The model under review builds one solid part; all positions refer to its coordinate system, in mm. A direction names the side the tool comes from. Round coordinates to 2 decimals unless told otherwise and drop trailing zeros. Write each loop counter-clockwise with the first axis right and the second up, starting at its lowest first coordinate (ties: lowest second). Pieces come first, ordered by that corner, then holes. Notation, with made-up numbers: (87, 80) - (117, 80) arc R28 cw to (117, 119) - close; hole circle Ø6 at (-32.5, 41.25). An arc over 180 degrees is marked (long way). Write each question's results on one line, items separated by ' | '.
```python
from build123d import *

# Parameters (mm, degrees)
SKETCH_1_R          = 5.5
EXTRUDE_1_DEPTH     = 37.5
SKETCH_2_R          = 4.25
CUT_EXTRUDE_1_DEPTH = 13
SKETCH_3_R          = 4.25
CUT_EXTRUDE_2_DEPTH = 101.822385015


with BuildPart() as part:
    # 草图1 → 凸台-拉伸1 (new, symmetric)
    with BuildSketch(Plane.XY):
        Polygon((0, 0), (80, 0), (80, 8), (64.335195596, 8), (51.148707324, 39.834998826), (62.225396744, 50.911688245), (56.568542495, 56.568542495), align=None)
        with Locations((22.17310878, 9.184402377)):
            Circle(SKETCH_1_R, mode=Mode.SUBTRACT)
        Polygon((7.242640687, 3), (15.457113006, 3), (13.279414953, 9.036774265), align=None, mode=Mode.SUBTRACT)
        with BuildLine():
            Line((29.347952769, 6), (61.91644612, 6))
            Line((61.91644612, 6), (48.024179606, 39.538898231))
            Line((48.024179606, 39.538898231), (24.994777104, 16.509495729))
            ThreePointArc((24.994777104, 16.509495729), (24.712781801, 15.655157608), (25.231380538, 14.919990739))
            ThreePointArc((25.231380538, 14.919990739), (28.178325742, 11.671844687), (28.391306903, 7.29125365))
            ThreePointArc((28.391306903, 7.29125365), (28.544443699, 6.404707488), (29.347952769, 6))
        make_face(mode=Mode.SUBTRACT)
    extrude(amount=EXTRUDE_1_DEPTH, both=True)

    # 草图2 → 切除-拉伸1 (cut)
    with BuildSketch(Plane(origin=(0, 0, 0), x_dir=(0, 0, 1), z_dir=(-0.7071067811865477, 0.7071067811865475, 0))):
        with Locations(Location((20, 70, 0), (0, 0, 270))):
            Circle(SKETCH_2_R)
        with Locations(Location((-20, 70, 0), (0, 0, 270))):
            Circle(SKETCH_2_R)
    extrude(amount=-CUT_EXTRUDE_1_DEPTH, mode=Mode.SUBTRACT)

    # 草图3 → 切除-拉伸2 (cut, through all)
    with BuildSketch(Plane(origin=(0, 8, 0), x_dir=(1, 0, 0), z_dir=(0, 1, 0))):
        with Locations(Location((70, -20, 0), (0, 0, 270))):
            Circle(SKETCH_3_R)
        with Locations(Location((70, 20, 0), (0, 0, 270))):
            Circle(SKETCH_3_R)
    extrude(amount=-CUT_EXTRUDE_2_DEPTH, mode=Mode.SUBTRACT)


solid = part.part
```
Q1. The part is to be moulded in two halves that separate along X. For faces 1 (the flat face through (14.38, 5.98, 0.52)), 2 (the flat face through (56.61, 45.296, 0.525)), 3 (the flat face through (34, 28, -37.5)), say which applies: released by +X, released by -X, zero draft, split by the parting line, or undercut.
Evaluation:
face 1: undercut | face 2: released by +X | face 3: zero draft
Q2. Insertion check: P1, Ø6.5, axis at x = 9.5, z = 12, coming from the +Y side; P2, Ø5, axis at x = 14, z = 1.5, coming from the +Y side; P3, Ø12, axis at y = 41, z = -10.5, coming from the +X side. Each pin has a flat end and moves straight along its axis. Give the tip position at first contact, or say it passes through.
Evaluation:
P1: stops at y = 12.75 | P2: stops at y = 16.5 | P3: stops at x = 58.31
Q3. We need section A-A (x = 70). State the section outline as (y, z) points, plus the area to 3 significant figures.
Evaluation:
outline: (0, -37.5) - (8, -37.5) - (8, -24.25) - (0, -24.25) - close; (0, -15.75) - (8, -15.75) - (8, 15.75) - (0, 15.75) - close; (0, 24.25) - (8, 24.25) - (8, 37.5) - (0, 37.5) - close | area: 464 mm^2
Q4. For probe 1 along X at (y, z) = (4.25, -20); probe 2 along Y at (x, z) = (56.5, -15); probe 3 along X at (y, z) = (5, 20), list the stretches that pass through material, from the lowest coordinate up.
Evaluation:
probe 1: x = 4.25 to 8.49, 15.01 to 19.74, 24.6 to 65.75, 74.25 to 80 | probe 2: y = 0 to 6, 19.08 to 26.92, 45.19 to 56.5 | probe 3: x = 5 to 9.24, 14.74 to 18.6, 25.74 to 65.75, 74.25 to 80
Q5. We need section C-C (y = 27.5). State the section outline as (x, z) points, plus the area to 3 significant figures.
Evaluation:
outline: (27.5, -37.5) - (35.99, -37.5) - (35.99, 37.5) - (27.5, 37.5) - close; (53.01, -37.5) - (56.26, -37.5) - (56.26, 37.5) - (53.01, 37.5) - close | area: 880 mm^2
Q6. Tool access review of faces 4 (the flat face through (80, 4, 1)), 5 (the flat face through (34, 28, 37.5)), 6 (the flat face through (72, 8, 1)), 7 (the flat face through (57.834, 23.695, 0.525)), 8 (the flat face through (11, 3, 1)): name each direction out of +Z, -Z, +X, -X, +Y, -Y from which nothing blocks a thin tool from reaching the whole face with its end or side.
Evaluation:
face 4: +Z, -Z, +X, +Y, -Y | face 5: +Z, +X, -X, +Y, -Y | face 6: +Z, -Z, +X, +Y | face 7: +Z, -Z, +X | face 8: +Z, -Z
Q7. We need section B-B (z = 20). State how many separate pieces and enclosed holes the cut face has, plus the area to 3 significant figures.
Evaluation:
separate pieces: 3 | enclosed holes: 3 | area: 873 mm^2
Q8. We need section D-D (x = 23). State the section outline as (y, z) points.
Evaluation:
outline: (0, -37.5) - (3.75, -37.5) - (3.75, 37.5) - (0, 37.5) - close; (14.62, -37.5) - (23, -37.5) - (23, 37.5) - (14.62, 37.5) - close
